Autodesk Inventor part; units mm, degrees
ref_plane "YZ Plane" through (0, 0, 0) normal (1, 0, 0) x (0, 1, 0)
ref_plane "XZ Plane" through (0, 0, 0) normal (0, 1, 0) x (-1, 0, 0)
ref_plane "XY Plane" through (0, 0, 0) normal (0, 0, 1) x (1, 0, 0)
sketch "Esboço1" plane through (0, 0, 0) normal (0, 0, 1) x (1, 0, 0)
  line L0 (-173, 38) -> (173, 38)
  line L1 (173, 38) -> (173, -38)
  line L2 (173, -38) -> (-173, -38)
  line L3 (-173, -38) -> (-173, 38)
  point P0 (0, 0)
  point P1 (173, 0)
  point P2 (0, 38)
  dimension "d0" = 346
  dimension "d1" = 76
extrude "Extrusão1" add sketch "Esboço1" along normal blind 4
sketch "Esboço2" plane through (0, 0, 4) normal (0, 0, 1) x (1, 0, 0)
  line L0 (-173, 38) -> (-173, -38)
  line L1 (-173, 13) -> (-165, 13)
  line L2 (-165, 13) -> (-165, -13)
  line L3 (-165, -13) -> (-173, -13)
  line L4 (-173, -13) -> (-173, 13)
  line L5 (173, 38) -> (-173, 38)
  circle A0 centre (-165, 13) radius 1
  circle A1 centre (-165, -13) radius 1
  point P0 (0, 0)
  dimension "d4" = 8
  dimension "d5" = 26
  dimension "d6" = 25
  dimension "d7" = 2
  dimension "d8" = 2
extrude "Extrusão2" cut sketch "Esboço2" against normal blind 10
mirror "Espelhamento1" about plane through (0, 0, 0) normal (1, 0, 0) of "Extrusão2"
sketch "Esboço3" plane through (0, 0, 0) normal (0, 0, -1) x (-1, 0, 0)
  line L0 (-113, -17) -> (-38, -17)
  line L1 (173, 38) -> (-173, 38)
  line L2 (-165, 12) -> (-165, -12)
  line L3 (-56, 23) -> (-110, 23)
  line L4 (-113, 20) -> (-113, 20)
  line L5 (-110, 17) -> (-56, 17)
  line L6 (-53, 20) -> (-53, 20)
  line L7 (-125, 12) -> (-41, 12)
  line L8 (-38, 9) -> (-38, 9)
  line L9 (-41, 6) -> (-125, 6)
  line L10 (-128, 9) -> (-128, 9)
  line L11 (-125, 0) -> (-41, 0)
  line L12 (-38, -3) -> (-38, -3)
  line L13 (-41, -6) -> (-125, -6)
  line L14 (-128, -3) -> (-128, -3)
  line L15 (-110, -17) -> (-56, -17)
  line L16 (-53, -14) -> (-53, -14)
  line L17 (-56, -11) -> (-110, -11)
  line L18 (-113, -14) -> (-113, -14)
  arc A0 (-113, -14) -> (-110, -17) centre (-110, -14) ccw
  arc A1 (-110, -11) -> (-113, -14) centre (-110, -14) ccw
  arc A2 (-56, -17) -> (-53, -14) centre (-56, -14) ccw
  arc A3 (-53, -14) -> (-56, -11) centre (-56, -14) ccw
  arc A4 (-38, -3) -> (-41, 0) centre (-41, -3) ccw
  arc A5 (-41, -6) -> (-38, -3) centre (-41, -3) ccw
  arc A6 (-41, 6) -> (-38, 9) centre (-41, 9) ccw
  arc A7 (-38, 9) -> (-41, 12) centre (-41, 9) ccw
  arc A8 (-56, 17) -> (-53, 20) centre (-56, 20) ccw
  arc A9 (-113, 20) -> (-110, 17) centre (-110, 20) ccw
  arc A10 (-110, 23) -> (-113, 20) centre (-110, 20) ccw
  arc A11 (-53, 20) -> (-56, 23) centre (-56, 20) ccw
  arc A12 (-128, -3) -> (-125, -6) centre (-125, -3) ccw
  arc A13 (-125, 0) -> (-128, -3) centre (-125, -3) ccw
  arc A14 (-128, 9) -> (-125, 6) centre (-125, 9) ccw
  arc A15 (-125, 12) -> (-128, 9) centre (-125, 9) ccw
  point P0 (0, 0)
  point P1 (-53, 23)
  point P2 (-38, 6)
  point P3 (-38, 12)
  point P4 (-38, -6)
  point P5 (-38, 0)
  point P6 (-53, -11)
  point P7 (-53, -17)
  dimension "d16" = 6
  dimension "d17" = 5
  dimension "d18" = 6
  dimension "d19" = 6
  dimension "d20" = 6
  dimension "d22" = 90
  dimension "d23" = 90
  dimension "d24" = 60
  dimension "d25" = 15
  dimension "d26" = 37
  dimension "d27" = 37
  dimension "d28" = 60
  dimension "d29" = 15
  dimension "d30" = 3
  dimension "d31" = 3
  dimension "d32" = 3
  dimension "d35" = 15
  dimension "d36" = 6
  dimension "d37" = 6
  dimension "d38" = 6
  dimension "d39" = 5
extrude "Extrusão3" cut sketch "Esboço3" against normal blind 10
mirror "Espelhamento2" about plane through (0, 0, 0) normal (1, 0, 0) of "Extrusão3"
properties part number "placa auto falante"
Verification items for the finished model (mm, model axes). Round coordinates to 2 decimals unless told otherwise and drop trailing zeros. Put each result on its own line as item: value. Start each with the question number.
(1) Section check A-A (z = 1.6). State how many separate pieces and enclosed holes the cut face has, then the cut area to 3 significant figures.
(2) Depth check by flat-ended pin: pin 1 Ø2 at (y, z) = (3, 2) entering from -X. Enter the tip coordinate at first touch or a pass-through.
(3) Material ranges on line 1 along X through (y, z) = (-3, 1.5); line 2 along Y through (x, z) = (69, 1.2); line 3 along Y through (x, z) = (39, 0.3), recorded low to high.
Completed:
1. separate pieces: 1
1. enclosed holes: 8
1. area: 22,300 mm2
2. pin 1: stops at x = -165
3. line 1: x = -165 to -128, -38 to 38, 128 to 165
3. line 2: y = -38 to -17, -11 to -6, 0 to 6, 12 to 17, 23 to 38
3. line 3: y = -38 to -5.24, -0.76 to 6.76, 11.24 to 38
